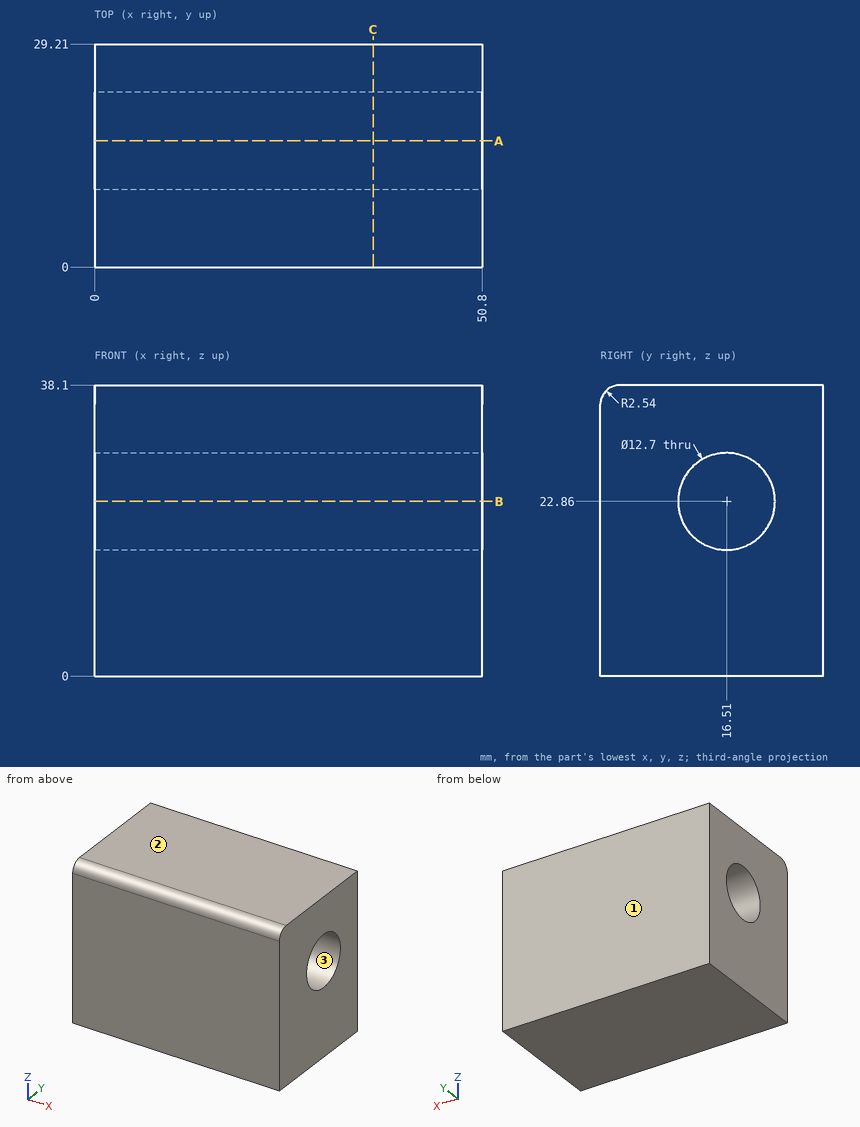
Study the drawing (mm; zero at the part's minimum x, y, z) and answer. Coordinates: 2 decimals unless noted, no trailing zeros. Loops run counter-clockwise (first coordinate to the right, second up) from the corner with the lowest first, then second, coordinate; pieces in that order, holes last. Notation, with made-up numbers: M 26,-12.5 L 72,-12.5 A26 ccw 72,15.5 Z; hole C 77,85 d11. An arc over 180 degrees is marked long. Answer in a Markdown table with one row per item. Add a question column.
1. Find section B-B, the plane z = 22.86. Write down the section's boundary in (x, y).
2. The mould has two halves that part along Y. Classify the marked faces 1, 2 and 3: pulls with the +Y half, pulls with the -Y half, needs draft (parallel to the pull), parting line crosses it, or undercut.
3. Consider L1, parallel to Z at x = 19, y = 16.51; L2, parallel to Y at x = 20, z = 20.5; L3, parallel to Z at x = 29.5, y = 11.5. Determine where each line is inside the solid, lowest interval first.
4. A flat-ended cylindrical pin translates along its axis: P1, Ø12, axis at y = 17, z = 31, coming from the -X side. Find the tip coordinate at first contact, or state that the pin passes through.
5. Find section C-C, the plane x = 36.5. Write down the section's boundary in (y, z), then the cut area to 3 significant figures.
6. Find section A-A, the plane y = 16.51. Write down the section's boundary in (x, z), then the cut area to 3 significant figures.
Reported:
| question | item | result |
|---|---|---|
| 1 | outline | M 0,0 L 50.8,0 L 50.8,10.16 L 0,10.16 Z; M 0,22.86 L 50.8,22.86 L 50.8,29.21 L 0,29.21 Z |
| 2 | face 1 | pulls with the +Y half |
| 2 | face 2 | needs draft |
| 2 | face 3 | undercut |
| 3 | L1 | z = 0 to 16.51, 29.21 to 38.1 |
| 3 | L2 | y = 0 to 10.61, 22.41 to 29.21 |
| 3 | L3 | z = 0 to 18.96, 26.76 to 38.1 |
| 4 | P1 | stops at x = 0 |
| 5 | outline | M 0,0 L 29.21,0 L 29.21,38.1 L 2.54,38.1 A2.54 ccw 0,35.56 Z; hole C 16.51,22.86 d12.7 |
| 5 | area | 985 mm^2 |
| 6 | outline | M 0,0 L 50.8,0 L 50.8,16.51 L 0,16.51 Z; M 0,29.21 L 50.8,29.21 L 50.8,38.1 L 0,38.1 Z |
| 6 | area | 1,290 mm^2 |
